from build123d import *

# Parameters (mm, degrees)
SKETCH1_W                = 10
SKETCH1_H                = 13.3
BOSS_EXTRUDE1_DEPTH      = 1
BOSS_EXTRUDE2_DEPTH      = 2.46
BOSS_EXTRUDE2_DEPTH_BACK = 3.34
SKETCH2_W                = 9
SKETCH2_H                = 7
SKETCH3_R                = 2.1
BOSS_EXTRUDE3_DEPTH      = 4.93
CHAMFER1_SIZE            = 2
CHAMFER1_SIZE2           = 0.3
BOSS_EXTRUDE4_DEPTH      = 1


with BuildPart() as part:
    # Sketch1 → Boss-Extrude1 (new body)
    with BuildSketch(Plane(origin=(0, 0, 0), x_dir=(1, 0, 0), z_dir=(0, 1, 0))):
        Rectangle(SKETCH1_W, SKETCH1_H)
    extrude(amount=BOSS_EXTRUDE1_DEPTH)

    # Sketch2 → Boss-Extrude2 (add, two sides: drawn at the far end of the back side and taken through both)
    with BuildSketch(Plane(origin=(0, 1, 0), x_dir=(1, 0, 0), z_dir=(0, 1, 0)).offset(-BOSS_EXTRUDE2_DEPTH_BACK)):
        Rectangle(SKETCH2_W, SKETCH2_H)
    extrude(amount=BOSS_EXTRUDE2_DEPTH + BOSS_EXTRUDE2_DEPTH_BACK)

    # Sketch3 → Boss-Extrude3 (add)
    with BuildSketch(Plane(origin=(0, 3.46, 0), x_dir=(1, 0, 0), z_dir=(0, 1, 0))):
        with Locations(Location((0, 0, 0), (0, 0, 270))):
            Circle(SKETCH3_R)
    extrude(amount=BOSS_EXTRUDE3_DEPTH)

    # Chamfer1
    chamfer1_edges = [part.edges().sort_by_distance(p)[0] for p in [
        (0, 8.39, -2.1),
    ]]
    chamfer1_side = [part.faces().sort_by_distance(p)[0] for p in [
        (0, 5.925, -2.1),
    ]]
    chamfer(chamfer1_edges, length=CHAMFER1_SIZE, length2=CHAMFER1_SIZE2, reference=chamfer1_side[0])

    # Sketch5 → Boss-Extrude4 (add)
    with BuildSketch(Plane.XY.offset(6.65)):
        Polygon((-4.31, 1), (-4.31, -3.34), (-4.04, -4.34), (-4.04, -10.21), (-3.58, -10.21), (-3.58, -4.34), (-3.31, -3.34), (-3.31, 1), align=None)
        Polygon((-1.77, 1), (-1.77, -3.34), (-1.5, -4.34), (-1.5, -10.21), (-1.04, -10.21), (-1.04, -4.34), (-0.77, -3.34), (-0.77, 1), align=None)
        Polygon((0.77, 1), (0.77, -3.34), (1.04, -4.34), (1.04, -10.21), (1.5, -10.21), (1.5, -4.34), (1.77, -3.34), (1.77, 1), align=None)
        Polygon((3.31, 1), (3.31, -3.34), (3.58, -4.34), (3.58, -10.21), (4.04, -10.21), (4.04, -4.34), (4.31, -3.34), (4.31, 1), align=None)
    boss_extrude4 = extrude(amount=-BOSS_EXTRUDE4_DEPTH)

    # Mirror1: Boss-Extrude4 across plane
    add(boss_extrude4.mirror(Plane.XY))


solid = part.part
Here's how the part is built. I have some questions about the finished solid (model axes, mm). A direction names the side the tool comes from. Round coordinates to 2 decimals unless told otherwise and drop trailing zeros. Loops run counter-clockwise (first coordinate to the right, second up) from the corner with the lowest first, then second, coordinate; pieces in that order, holes last.
1. For P1, Ø1.1, axis at y = -6.5, z = 6, coming from the -X side; P2, Ø3, axis at x = -3.5, y = 3.5, coming from the -Z side; P3, Ø3, axis at x = 0, z = -1.5, coming from the -Y side, each with a flat end and sliding along its axis, tell me the tip position at first contact or that it passes through.
Answer list:
P1: stops at x = -4.04
P2: stops at z = -3.5
P3: stops at y = -2.34
2. If we section it at B-B on z = 0: Write out the boundary of the cut face in (x, y).
Answer list:
outline: (-5, 0) - (-4.5, 0) - (-4.5, -2.34) - (4.5, -2.34) - (4.5, 0) - (5, 0) - (5, 1) - (4.5, 1) - (4.5, 3.46) - (2.1, 3.46) - (2.1, 6.39) - (1.8, 8.39) - (-1.8, 8.39) - (-2.1, 6.39) - (-2.1, 3.46) - (-4.5, 3.46) - (-4.5, 1) - (-5, 1) - close
3. We'd pull the mould along X, two halves only. Please class faces 1 (the face through (3.58, -7, -6)), 2 (the face through (4.5, 2, 0)), 3 (the face through (0, 2, -3.5)), 4 (the face through (-1.77, -2, -6)): +X half, -X half, draft (parallel to the pull), parting line (faces both ways), or undercut.
Answer list:
face 1: undercut
face 2: +X half
face 3: draft
face 4: undercut
4. Which directions (+Z, -Z, +X, -X, +Y, -Y) give clear straight access to the entire face, cutting with the end or side of a thin tool? Please do faces 5 (the face through (-1.04, -7, 6)), 6 (the face through (1.77, -2, 6)), 7 (the face through (0.631, 4.904, 2.003)), 8 (the face through (4.31, -2, 6)).
Answer list:
face 5: +Z, -Z, -Y
face 6: +Z, -Y
face 7: +Y
face 8: +Z, +X, -Y
5. If we section it at C-C on x = 0: Write out the boundary of the cut face in (y, z), plus the area to 3 significant figures.
Answer list:
outline: (-2.34, -3.5) - (0, -3.5) - (0, -6.65) - (1, -6.65) - (1, -3.5) - (3.46, -3.5) - (3.46, -2.1) - (6.39, -2.1) - (8.39, -1.8) - (8.39, 1.8) - (6.39, 2.1) - (3.46, 2.1) - (3.46, 3.5) - (1, 3.5) - (1, 6.65) - (0, 6.65) - (0, 3.5) - (-2.34, 3.5) - close
area: 67.0 mm2
6. If I drill on line 1 along Y through (x, z) = (-3, -1); line 2 along Y through (x, z) = (3.5, 4.5); line 3 along Z through (x, y) = (0.5, -0.5), over which ranges is the centre line in solid material (lowest first)?
Answer list:
line 1: y = -2.34 to 3.46
line 2: y = 0 to 1
line 3: z = -3.5 to 3.5
7. If we section it at A-A on y = -9: Count the separate pieces of the cut face and the enclosed holes in it, plus the area to 3 significant figures.
Answer list:
separate pieces: 8
enclosed holes: 0
area: 3.68 mm2
